Check sheet for the drawn part. Datum: minimum x, y, z corner. Units: mm. A direction names the side the tool comes from. Round coordinates to 2 decimals unless told otherwise and drop trailing zeros. Order: outer loops, then holes, each group sorted by start corner. A loop starts at its lowest first (then second) coordinate and runs counter-clockwise, first axis right, second up. Notation, with made-up numbers: M 68.25,-22.75 L 100.25,-22.75 A13 cw 100.25,-6.75 Z; hole C 84,1 d11. An arc over 180 degrees is marked long. Use one line per item in the form item = value. Start each with the question number.
Item 1: Cross-section at B-B on z = 1.5. Enter the section's corners in (x, y) (1 decimal), then the cut area to 3 significant figures.
Item 2: Go/stop test with flat-tipped pins: pin 1 Ø4 at (y, z) = (6.5, 3) entering from +X; pin 2 Ø1.3 at (y, z) = (1, 3) entering from -X; pin 3 Ø1.5 at (y, z) = (6, 6.5) entering from +X; pin 4 Ø1.4 at (y, z) = (3.5, 2.5) entering from -X. Record where each tip stops, or that it passes through.
Item 3: Thickness scan on probe 1 along Y at (x, z) = (11.25, 2.25); probe 2 along Y at (x, z) = (3.25, 1.5) (1 decimal); probe 3 along Z at (x, y) = (6.75, 12) (1 decimal). Record the ranges inside material, lowest first. Write a range as [from, to].
Item 4: Cross-section at C-C on y = 5.25. Enter the section's corners in (x, z) (1 decimal).
Item 5: Cross-section at A-A on x = 3. Enter the section's corners in (y, z) (1 decimal).
Item 6: Release check for a two-part mould opening along Y. For the marked faces 5, 6, 7 and 8 record: +Y half, -Y half, draft (parallel to the pull), parting line (faces both ways), or undercut.
Item 7: Cross-section at D-D on x = 6. Enter the section's corners in (y, z) (1 decimal).
Item 8: Tool access check on the marked faces 1, 2, 3 and 4. Record the directions out of +Z, -Z, +X, -X, +Y, -Y that give a thin tool (end or side, any length) a straight path to the whole face; none if there is none.
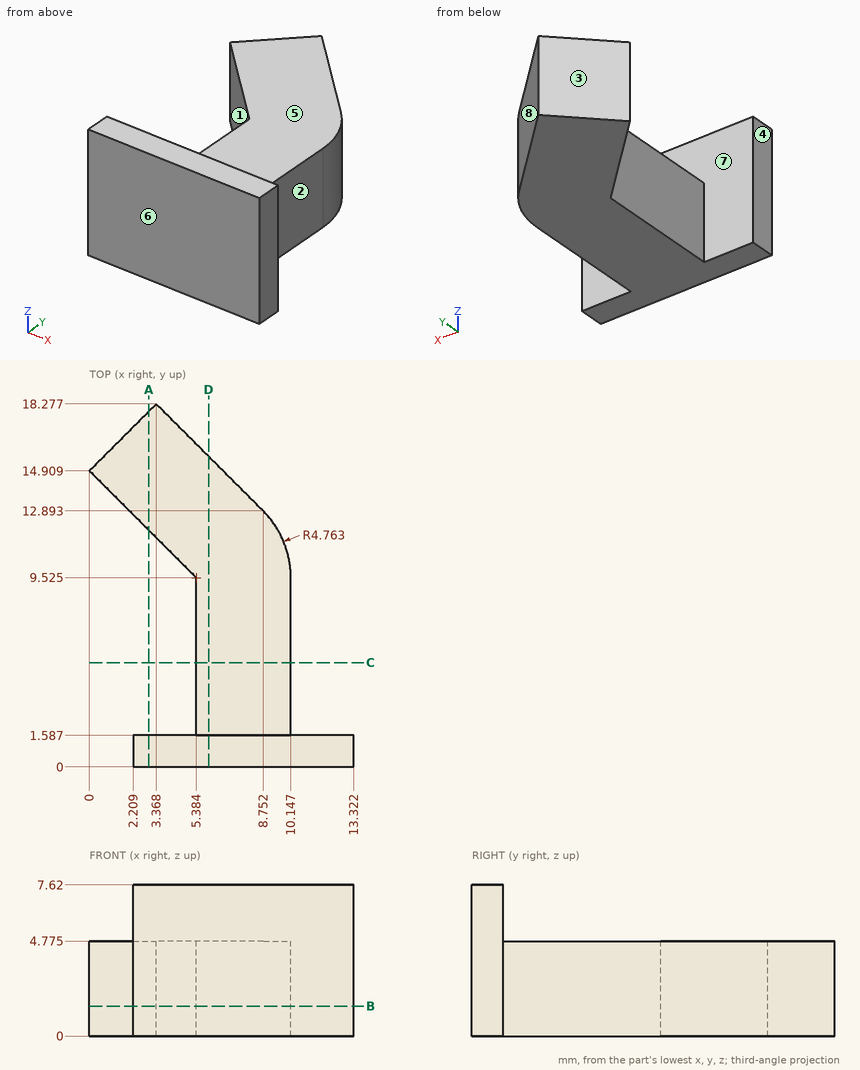
Output values:
q1.outline = M 0,14.9 L 5.4,9.5 L 5.4,1.6 L 2.2,1.6 L 2.2,0 L 13.3,0 L 13.3,1.6 L 10.1,1.6 L 10.1,9.5 A4.8 ccw 8.8,12.9 L 3.4,18.3 Z
q1.area = 101 mm2
q2.pin_1 = 10.15
q2.pin_2 = 2.21
q2.pin_3 = through
q2.pin_4 = 5.38
q3.probe_1 = [0, 1.59]
q3.probe_2 = [0, 1.6], [11.7, 18.2]
q3.probe_3 = [0, 4.8]
q4.outline = M 5.4,0 L 10.1,0 L 10.1,4.8 L 5.4,4.8 Z
q5.outline = M 0,0 L 1.6,0 L 1.6,7.6 L 0,7.6 Z; M 11.9,0 L 17.9,0 L 17.9,4.8 L 11.9,4.8 Z
q6.face_5 = draft
q6.face_6 = -Y half
q6.face_7 = undercut
q6.face_8 = +Y half
q7.outline = M 0,0 L 15.6,0 L 15.6,4.8 L 1.6,4.8 L 1.6,7.6 L 0,7.6 Z
q8.face_1 = +Z, -Z, -X
q8.face_2 = +Z, -Z, +X, +Y
q8.face_3 = +Z, -Z, -X, +Y
q8.face_4 = +Z, -Z, -X, -Y
